Answer from the drawing. Dimensions are ordinates in mm from the lowest x, y and z of the part. Give positions to 0.01 mm unless a question says otherwise; leave off trailing zeros. Loops run counter-clockwise (first coordinate to the right, second up) from the corner with the lowest first, then second, coordinate; pieces in that order, holes last. Notation, with made-up numbers: (-15.5, -1.5) - (-11.5, -1.5) arc R19 ccw to (-11.5, 2.5) - close; hole circle Ø10 at (-2, 20). An arc over 180 degrees is marked (long way). One line per item, written item: value.
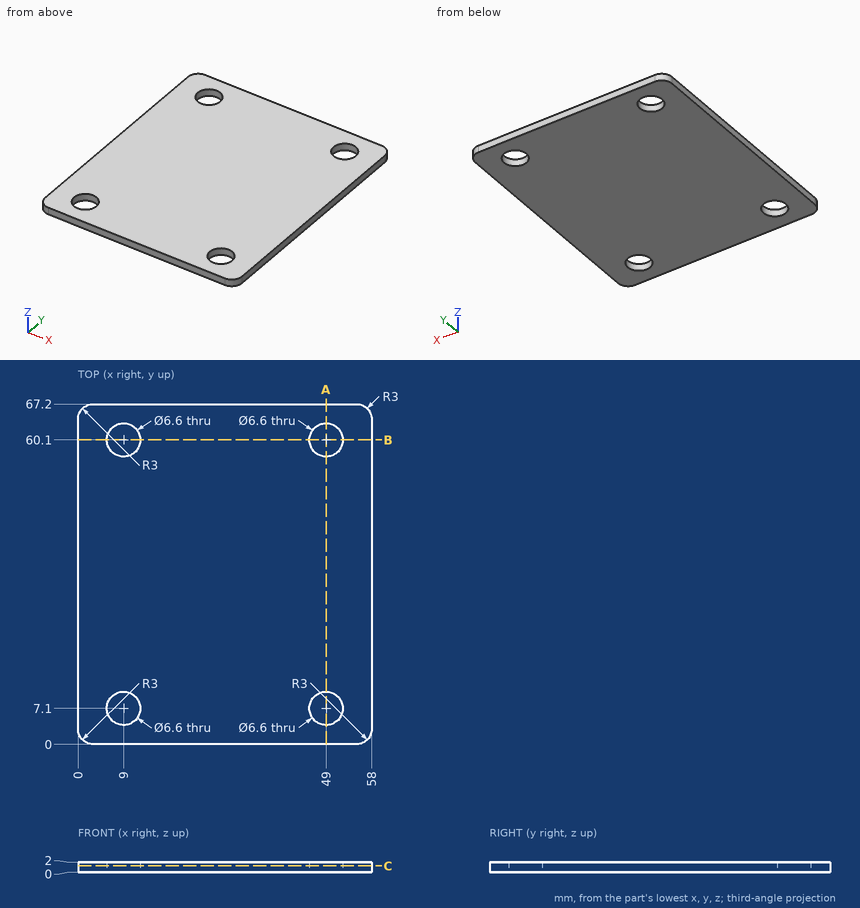
1. Find the intervals of material crossed by line 1 along Y through (x, z) = (49, 1), in increasing order.
Output:
line 1: y = 0 to 3.8, 10.4 to 56.8, 63.4 to 67.2
2. Section A-A (x = 49) is taken. Write down the section's boundary in (y, z).
Output:
outline: (0, 0) - (3.8, 0) - (3.8, 2) - (0, 2) - close; (10.4, 0) - (56.8, 0) - (56.8, 2) - (10.4, 2) - close; (63.4, 0) - (67.2, 0) - (67.2, 2) - (63.4, 2) - close
3. Section B-B (y = 60.1) is taken. Write down the section's boundary in (x, z).
Output:
outline: (0, 0) - (5.7, 0) - (5.7, 2) - (0, 2) - close; (12.3, 0) - (45.7, 0) - (45.7, 2) - (12.3, 2) - close; (52.3, 0) - (58, 0) - (58, 2) - (52.3, 2) - close
4. Flat-ended cylindrical pins translate along their axes: pin 1 Ø12 at (x, y) = (10, 50.5) entering from -Z; pin 2 Ø4 at (x, y) = (49, 7.1) entering from +Z. Find the tip coordinate at first contact, or state that the pin passes through.
Output:
pin 1: stops at z = 0
pin 2: passes through
5. Section C-C (z = 1.3) is taken. Write down the section's boundary in (x, y), and give its area (3 significant figures).
Output:
outline: (0, 3) arc R3 ccw to (3, 0) - (55, 0) arc R3 ccw to (58, 3) - (58, 64.2) arc R3 ccw to (55, 67.2) - (3, 67.2) arc R3 ccw to (0, 64.2) - close; hole circle Ø6.6 at (9, 7.1); hole circle Ø6.6 at (9, 60.1); hole circle Ø6.6 at (49, 7.1); hole circle Ø6.6 at (49, 60.1)
area: 3,750 mm²
